Geometry: see drawing. Coordinates: mm, zero at the bounding-box minimum. Give positions to 0.01 mm unless a question says otherwise; leave off trailing zeros. Loops run counter-clockwise (first coordinate to the right, second up) from the corner with the lowest first, then second, coordinate; pieces in that order, holes last. Notation, with made-up numbers: M 2.25,-13 L 8.25,-13 A12 cw 8.25,2 Z; hole C 57.5,82 d1. An arc over 180 degrees is marked long. Put each result on its own line as item: value.
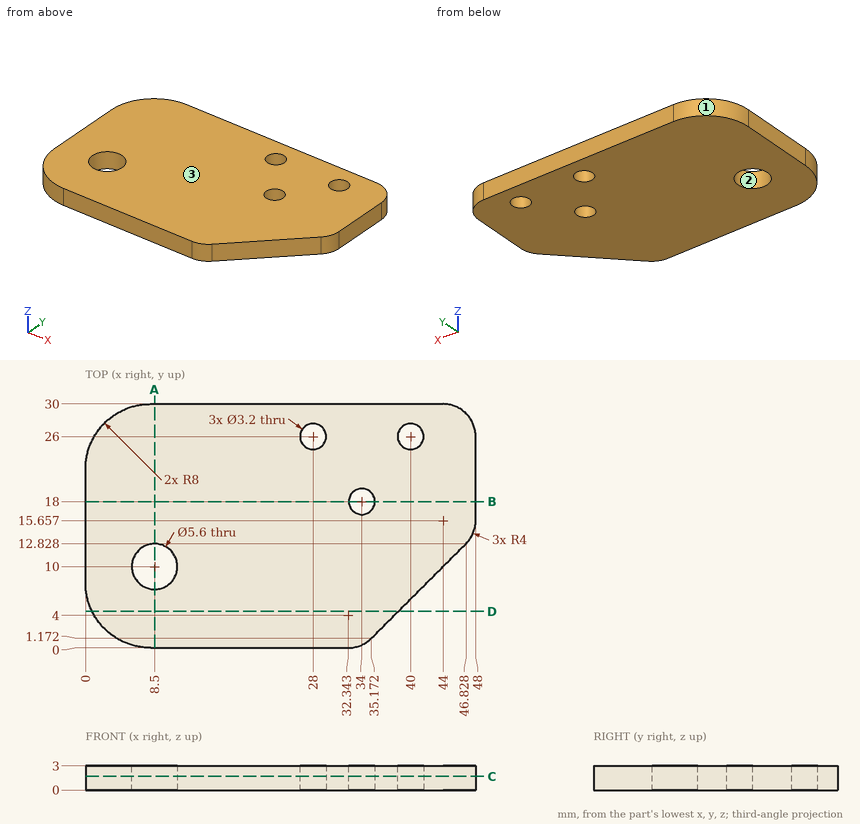
1. Contact query for flat-ended pins moving along their axis: P1, Ø1, axis at y = 9, z = 0.5, coming from the +X side; P2, Ø1, axis at y = 11, z = 2.5, coming from the +X side. Output: stop coordinate, or through.
Found:
P1: x = 43.5
P2: x = 45.5
2. Section query D-D (y = 4.5). Output: boundary loops of the cut face in (x, z).
Found:
outline: M 0.81,0 L 38.5,0 L 38.5,3 L 0.81,3 Z
3. Section query C-C (z = 1.7). Output: boundary loops of the cut face in (x, y), plus the area to 3 significant figures.
Found:
outline: M 0,8 A8 ccw 8,0 L 32.34,0 A4 ccw 35.17,1.17 L 46.83,12.83 A4 ccw 48,15.66 L 48,26 A4 ccw 44,30 L 8,30 A8 ccw 0,22 Z; hole C 8.5,10 d5.6; hole C 28,26 d3.2; hole C 34,18 d3.2; hole C 40,26 d3.2
area: 1,260 mm^2
4. Material intervals for line 1 (Y direction, x = 8.5, z = 1.4); line 2 (X direction, y = 26, z = 1); line 3 (X direction, y = 25.25, z = 1.2) (1 decimal), sorted ascending. Write a range as from..to.
Found:
line 1: 0..7.2, 12.8..30
line 2: 1.07..26.4, 29.6..38.4, 41.6..48
line 3: 0.7..26.6, 29.4..38.6, 41.4..48
5. Section query B-B (y = 18). Output: boundary loops of the cut face in (x, z).
Found:
outline: M 0,0 L 32.4,0 L 32.4,3 L 0,3 Z; M 35.6,0 L 48,0 L 48,3 L 35.6,3 Z
6. Draft query along X for the marked faces 1, 2 and 3. Return one class per face: pulls with the +X half, pulls with the -X half, needs draft (parallel to the pull), parting line crosses it, or undercut.
Found:
face 1: pulls with the -X half
face 2: undercut
face 3: needs draft
7. Section query A-A (x = 8.5). Output: boundary loops of the cut face in (y, z).
Found:
outline: M 0,0 L 7.2,0 L 7.2,3 L 0,3 Z; M 12.8,0 L 30,0 L 30,3 L 12.8,3 Z
